Autodesk Inventor part; units mm, degrees
ref_plane "YZ Plane" through (0, 0, 0) normal (1, 0, 0) x (0, 1, 0)
ref_plane "XZ Plane" through (0, 0, 0) normal (0, 1, 0) x (-1, 0, 0)
ref_plane "XY Plane" through (0, 0, 0) normal (0, 0, 1) x (1, 0, 0)
sketch "Sketch1" plane through (0, 0, 0) normal (0, 0, 1) x (1, 0, 0)
  arc A0 (-3.1269, -1.4516) -> (-2.9447, -0.6532) centre (-10.144, 0.57) ccw
  arc A1 (-2.9447, -0.6532) -> (0, 0) centre (-4.7545, 14.4689) ccw
  line L0 (0, 0) -> (0, 1.1399)
  arc A2 (0, 1.1399) -> (-2.9447, 1.7932) centre (-4.7545, -13.329) ccw
  arc A3 (-2.9447, 1.7932) -> (-3.1269, 2.5916) centre (-10.144, 0.57) ccw
  arc A4 (-3.1269, 2.5916) -> (-0.7573, 4.4578) centre (-11.3188, 15.4309) ccw
  line L1 (-0.7573, 4.4578) -> (-1.2519, 5.4848)
  arc A5 (-1.2519, 5.4848) -> (-4.1884, 4.7957) centre (0.7423, -9.6141) ccw
  arc A6 (-4.1884, 4.7957) -> (-4.699, 5.436) centre (-10.144, 0.57) ccw
  arc A7 (-4.699, 5.436) -> (-3.3737, 8.1455) centre (-17.6504, 13.4495) ccw
  line L2 (-3.3737, 8.1455) -> (-4.265, 8.8563)
  arc A8 (-4.265, 8.8563) -> (-6.6117, 6.9613) centre (4.0829, -3.8822) ccw
  arc A9 (-6.6117, 6.9613) -> (-7.3495, 7.3166) centre (-10.144, 0.57) ccw
  arc A10 (-7.3495, 7.3166) -> (-7.3311, 10.3328) centre (-22.4952, 8.9171) ccw
  line L3 (-7.3311, 10.3328) -> (-8.4425, 10.5865)
  arc A11 (-8.4425, 10.5865) -> (-9.7346, 7.861) centre (4.6057, 2.7315) ccw
  arc A12 (-9.7346, 7.861) -> (-10.5535, 7.861) centre (-10.144, 0.57) ccw
  arc A13 (-10.5535, 7.861) -> (-11.8456, 10.5865) centre (-24.8938, 2.7315) ccw
  line L4 (-11.8456, 10.5865) -> (-12.957, 10.3328)
  arc A14 (-12.957, 10.3328) -> (-12.9386, 7.3166) centre (2.2072, 8.9171) ccw
  arc A15 (-12.9386, 7.3166) -> (-13.6764, 6.9613) centre (-10.144, 0.57) ccw
  arc A16 (-13.6764, 6.9613) -> (-16.0231, 8.8563) centre (-24.371, -3.8822) ccw
  line L5 (-16.0231, 8.8563) -> (-16.9143, 8.1455)
  arc A17 (-16.9143, 8.1455) -> (-15.5891, 5.436) centre (-2.6377, 13.4495) ccw
  arc A18 (-15.5891, 5.436) -> (-16.0997, 4.7957) centre (-10.144, 0.57) ccw
  arc A19 (-16.0997, 4.7957) -> (-19.0362, 5.4848) centre (-21.0303, -9.6141) ccw
  line L6 (-19.0362, 5.4848) -> (-19.5308, 4.4578)
  arc A20 (-19.5308, 4.4578) -> (-17.1611, 2.5916) centre (-8.9693, 15.4309) ccw
  arc A21 (-17.1611, 2.5916) -> (-17.3433, 1.7932) centre (-10.144, 0.57) ccw
  arc A22 (-17.3433, 1.7932) -> (-20.288, 1.1399) centre (-15.5335, -13.329) ccw
  line L7 (-20.288, 1.1399) -> (-20.288, 0)
  arc A23 (-20.288, 0) -> (-17.3433, -0.6532) centre (-15.5335, 14.4689) ccw
  arc A24 (-17.3433, -0.6532) -> (-17.1611, -1.4516) centre (-10.144, 0.57) ccw
  arc A25 (-17.1611, -1.4516) -> (-19.5308, -3.3178) centre (-8.9693, -14.291) ccw
  line L8 (-19.5308, -3.3178) -> (-19.0362, -4.3449)
  arc A26 (-19.0362, -4.3449) -> (-16.0997, -3.6558) centre (-21.0303, 10.7541) ccw
  arc A27 (-16.0997, -3.6558) -> (-15.5891, -4.296) centre (-10.144, 0.57) ccw
  arc A28 (-15.5891, -4.296) -> (-16.9143, -7.0056) centre (-2.6377, -12.3096) ccw
  line L9 (-16.9143, -7.0056) -> (-16.0231, -7.7163)
  arc A29 (-16.0231, -7.7163) -> (-13.6764, -5.8213) centre (-24.371, 5.0222) ccw
  arc A30 (-13.6764, -5.8213) -> (-12.9386, -6.1767) centre (-10.144, 0.57) ccw
  arc A31 (-12.9386, -6.1767) -> (-12.957, -9.1929) centre (2.2072, -7.7772) ccw
  line L10 (-12.957, -9.1929) -> (-11.8456, -9.4465)
  arc A32 (-11.8456, -9.4465) -> (-10.5535, -6.721) centre (-24.8938, -1.5916) ccw
  arc A33 (-10.5535, -6.721) -> (-9.7346, -6.721) centre (-10.144, 0.57) ccw
  arc A34 (-9.7346, -6.721) -> (-8.4425, -9.4465) centre (4.6057, -1.5916) ccw
  line L11 (-8.4425, -9.4465) -> (-7.3311, -9.1929)
  arc A35 (-7.3311, -9.1929) -> (-7.3495, -6.1767) centre (-22.4952, -7.7772) ccw
  arc A36 (-7.3495, -6.1767) -> (-6.6117, -5.8213) centre (-10.144, 0.57) ccw
  arc A37 (-6.6117, -5.8213) -> (-4.265, -7.7163) centre (4.0829, 5.0222) ccw
  line L12 (-4.265, -7.7163) -> (-3.3737, -7.0056)
  arc A38 (-3.3737, -7.0056) -> (-4.699, -4.296) centre (-17.6504, -12.3096) ccw
  arc A39 (-4.699, -4.296) -> (-4.1884, -3.6558) centre (-10.144, 0.57) ccw
  arc A40 (-4.1884, -3.6558) -> (-1.2519, -4.3449) centre (0.7423, 10.7541) ccw
  line L13 (-1.2519, -4.3449) -> (-0.7573, -3.3178)
  arc A41 (-0.7573, -3.3178) -> (-3.1269, -1.4516) centre (-11.3188, -14.291) ccw
  line L14 (-9.144, 5.57) -> (-11.144, 5.57)
  line L15 (-9.144, 4.443) -> (-9.144, 5.57)
  arc A42 (-11.144, 4.443) -> (-9.144, 4.443) centre (-10.144, 0.57) ccw
  line L16 (-11.144, 5.57) -> (-11.144, 4.443)
extrude "Extrusion1" add sketch "Sketch1" against normal blind 13.208
chamfer "Chamfer1" distance 0.508 angle 45 2 edges at (-10.144, -3.43, 0) (-10.144, -3.43, -13.208)
properties part number "am-0741"
Work out the finished part from the listing and answer in its coordinate system (mm). A direction names the side the tool comes from. Give positions to 0.01 mm unless a question says otherwise; leave off trailing zeros. Write each loop counter-clockwise with the first axis right and the second up, starting at its lowest first coordinate (ties: lowest second). Pieces come first, ordered by that corner, then holes.
(1) Straight lines are drawn through the part: line 1 (X direction, y = 0.57, z = -9.5); line 2 (Y direction, x = -2.5, z = -1); line 3 (Y direction, x = -4, z = -5) (3 decimals). For each, find the intervals that lie inside material, in ascending order.
Final values:
line 1: x = -20.29 to -14.14, -6.14 to 0
line 2: y = -4.13 to -1.87, -0.59 to 1.73, 3.01 to 5.27
line 3: y = -7.505 to -5.555, -3.719 to 4.859, 6.695 to 8.645
(2) Which of the six approach directions +Z, -Z, +X, -X, +Y, -Y give full straight-line access (tool end or side, diameter ignored) to faces 5 (the cylindrical face through (-18.853, -0.395, -6.512)), 6 (the cylindrical face through (-13.023, -7.663, -6.512)), 7 (the cylindrical face through (-11.123, 9.237, -6.512)), 8 (the cylindrical face through (-1.912, 3.453, -6.512))?
Final values:
face 5: +Z, -Z, -X
face 6: +Z, -Z
face 7: +Z, -Z, +Y
face 8: +Z, -Z, +X
(3) The part is cut by section B-B on x = -2.5. Write down the section's boundary in (y, z), plus the area to 3 significant figures.
Final values:
outline: (-4.13, -13.21) - (-1.87, -13.21) - (-1.87, 0) - (-4.13, 0) - close; (-0.59, -13.21) - (1.73, -13.21) - (1.73, 0) - (-0.59, 0) - close; (3.01, -13.21) - (5.27, -13.21) - (5.27, 0) - (3.01, 0) - close
area: 90.2 mm2
(4) Flat-ended cylindrical pins translate along their axes: pin 1 Ø4 at (y, z) = (-2.5, -1.5) entering from +X; pin 2 Ø2 at (x, y) = (-10, -2.5) entering from -Z; pin 3 Ø4 at (x, z) = (-9, -10.5) entering from +Y. Find the tip coordinate at first contact, or state that the pin passes through.
Final values:
pin 1: stops at x = -0.76
pin 2: stops at z = -12.77
pin 3: stops at y = 10.59
(5) The part is cut by section A-A on y = 0.57. Write down the section's boundary in (x, z).
Final values:
outline: (-20.29, -13.21) - (-14.65, -13.21) - (-14.14, -12.7) - (-14.14, -0.51) - (-14.65, 0) - (-20.29, 0) - close; (-6.14, -12.7) - (-5.64, -13.21) - (0, -13.21) - (0, 0) - (-5.64, 0) - (-6.14, -0.51) - close
(6) The part is cut by section C-C on x = -5. Write down the section's boundary in (y, z), plus the area to 3 significant figures.
Final values:
outline: (-7.2, -13.21) - (8.34, -13.21) - (8.34, 0) - (-7.2, 0) - close
area: 205 mm2
(7) The part is cut by section D-D on x = -18. Write down the section's boundary in (y, z).
Final values:
outline: (-4.17, -13.21) - (-2.03, -13.21) - (-2.03, 0) - (-4.17, 0) - close; (-0.56, -13.21) - (1.7, -13.21) - (1.7, 0) - (-0.56, 0) - close; (3.17, -13.21) - (5.31, -13.21) - (5.31, 0) - (3.17, 0) - close
(8) The mould has two halves that part along Y. Classify faces 1 (the cylindrical face through (-18.811, 1.544, -6.512)), 2 (the cylindrical face through (-3.98, 6.74, -6.51)), 3 (the flat face through (-1.01, -3.84, -6.51)), 4 (the flat face through (-15, 1, -13.208)): pulls with the +Y half, pulls with the -Y half, needs draft (parallel to the pull), parting line crosses it, or undercut.
Final values:
face 1: undercut
face 2: undercut
face 3: pulls with the -Y half
face 4: needs draft
